```python
from build123d import *

# Parameters (mm, degrees)
SKETCH_W      = 43.2
SKETCH_H      = 70.2
PAD_DEPTH     = 1.6
SKETCH007_R   = 1.75
POCKET_DEPTH  = 1.6
SKETCH008_W   = 11.4
SKETCH008_H   = 1.6
PAD001_DEPTH  = 8
SKETCH009_W   = 1.6
SKETCH009_H   = 21.9
SKETCH009_H_2 = 26.9
PAD002_DEPTH  = 15
SKETCH010_R   = 2
PAD003_DEPTH  = 8.6


with BuildPart() as part:
    # Sketch → Pad (new body)
    with BuildSketch(Plane.XY):
        with Locations((21.6, 35.1)):
            Rectangle(SKETCH_W, SKETCH_H)
    extrude(amount=PAD_DEPTH)

    # Sketch007 (on Face6 of Pad) → Pocket (cut)
    with BuildSketch(Plane.XY.offset(1.6)):
        with Locations((4.6, 4.6)):
            Circle(SKETCH007_R)
        with Locations((38.6, 4.6)):
            Circle(SKETCH007_R)
        with Locations((4.6, 65.6)):
            Circle(SKETCH007_R)
        with Locations((38.6, 65.6)):
            Circle(SKETCH007_R)
    extrude(amount=-POCKET_DEPTH, mode=Mode.SUBTRACT)

    # Sketch008 (on Face5 of Pocket) → Pad001 (join)
    with BuildSketch(Plane.XY.offset(1.6)):
        with Locations((21.6, 0.8)):
            Rectangle(SKETCH008_W, SKETCH008_H)
    extrude(amount=PAD001_DEPTH)

    # Sketch009 (on Face5 of Pad001) → Pad002 (join)
    with BuildSketch(Plane.XY.offset(1.6)):
        with Locations((0.8, 42.75)):
            Rectangle(SKETCH009_W, SKETCH009_H)
        with Locations((42.4, 40.25)):
            Rectangle(SKETCH009_W, SKETCH009_H_2)
    extrude(amount=PAD002_DEPTH)

    # Sketch010 (on Face5 of Pad002) → Pad003 (join)
    with BuildSketch(Plane.XY.offset(1.6)):
        with Locations((21.6, 42)):
            Circle(SKETCH010_R)
        with Locations((21.6, 7)):
            Circle(SKETCH010_R)
    extrude(amount=PAD003_DEPTH)


solid = part.part
```
Verification items for the finished model (mm, model axes). A direction names the side the tool comes from. Coordinates: 2 decimals unless noted, no trailing zeros. Write each loop counter-clockwise with the first axis right and the second up, starting at its lowest first coordinate (ties: lowest second). Pieces come first, ordered by that corner, then holes. Notation, with made-up numbers: M 80.25,-20 L 111.25,-20 A7 cw 111.25,-16 Z; hole C 52.5,71 d9. An arc over 180 degrees is marked long. Answer as a JSON object with one key per item and string values. Group by question number.
(1) Cross-section at D-D, the plane y = 66.5. Record the cut outline in (x, z), and give its area (3 significant figures).
(2) Release check for a two-part mould opening along Y. For faces 4 (the face through (1, 53.7, 9)), 5 (the face through (21, 36, 0)), 6 (the face through (22, 1.6, 6)) record: +Y half, -Y half, draft (parallel to the pull), parting line (faces both ways), or undercut.
(3) Gauge pin test, flat ends, axial feed: pin 1 (3 mm diameter, centred on x = 22, y = 6.5, fed in from +Z); pin 2 (0.5 mm diameter, centred on x = 42.5, z = 10, fed in from +Y); pin 3 (0.8 mm diameter, centred on y = 1, z = 4, fed in from +X). Record the tip position at first contact, or that the pin passes through.
(4) Cross-section at B-B, the plane x = 38.6. Record the cut outline in (y, z).
(5) Cross-section at A-A, the plane z = 8.25. Record the cut outline in (x, y).
(6) Cross-section at C-C, the plane y = 38.5. Record the cut outline in (x, z).
(7) Tool access check on faces 1 (the face through (42, 53.7, 9)), 2 (the face through (42, 26.8, 9)), 3 (the face through (22, 42, 10.2)). Record the directions out of +Z, -Z, +X, -X, +Y, -Y that give a thin tool (end or side, any length) a straight path to the whole face; none if there is none.
(8) Material ranges on line 1 (Y direction, x = 4.6, z = 0.95); line 2 (X direction, y = 65.6, z = 0.85); line 3 (X direction, y = 33.5, z = 5.25), recorded low to high.
Reply:
{
 "1": {"outline": "M 0,0 L 3.1,0 L 3.1,1.6 L 0,1.6 Z; M 6.1,0 L 37.1,0 L 37.1,1.6 L 6.1,1.6 Z; M 40.1,0 L 43.2,0 L 43.2,1.6 L 40.1,1.6 Z", "area": "59.5 mm²"},
 "2": {"face 4": "+Y half", "face 5": "draft", "face 6": "undercut"},
 "3": {"pin 1": "z = 10.2", "pin 2": "y = 53.7", "pin 3": "x = 27.3"},
 "4": {"outline": "M 0,0 L 2.85,0 L 2.85,1.6 L 0,1.6 Z; M 6.35,0 L 63.85,0 L 63.85,1.6 L 6.35,1.6 Z; M 67.35,0 L 70.2,0 L 70.2,1.6 L 67.35,1.6 Z"},
 "5": {"outline": "M 0,31.8 L 1.6,31.8 L 1.6,53.7 L 0,53.7 Z; M 15.9,0 L 27.3,0 L 27.3,1.6 L 15.9,1.6 Z; C 21.6,7 d4; C 21.6,42 d4; M 41.6,26.8 L 43.2,26.8 L 43.2,53.7 L 41.6,53.7 Z"},
 "6": {"outline": "M 0,0 L 43.2,0 L 43.2,16.6 L 41.6,16.6 L 41.6,1.6 L 1.6,1.6 L 1.6,16.6 L 0,16.6 Z"},
 "7": {"face 1": "+Z, +X, -X, +Y", "face 2": "+Z, +X, -X, -Y", "face 3": "+Z, +Y, -Y"},
 "8": {"line 1": "0 to 2.85, 6.35 to 63.85, 67.35 to 70.2", "line 2": "0 to 2.85, 6.35 to 36.85, 40.35 to 43.2", "line 3": "0 to 1.6, 41.6 to 43.2"}
}
